Can you work these out from the model? Positions are in its coordinate system, mm. A direction names the side the tool comes from. Round coordinates to 2 decimals unless told otherwise and drop trailing zeros. Loops run counter-clockwise (first coordinate to the right, second up) from the corner with the lowest first, then second, coordinate; pieces in that order, holes last. Notation, with made-up numbers: M 42.5,53 L 65.5,53 A14 ccw 65.5,69 Z; hole C -37.5,29.5 d4. An arc over 180 degrees is marked long. Return JSON: item names as keys, results as strings.
```python
from build123d import *

# Parameters (mm, degrees)
ESQUISSE1_W             = 20
ESQUISSE1_H             = 80
ESQUISSE1_R             = 2.75
BOSS_EXTRU_1_DEPTH      = 5
BOSS_EXTRU_2_DEPTH      = 5
ESQUISSE4_R             = 2.75
BOSS_EXTRU_3_DEPTH      = 25
BOSS_EXTRU_4_DEPTH      = 20
ENL_V_MAT_EXTRU_1_REACH = 78.988
ESQUISSE6_R             = 6
ENL_V_MAT_EXTRU_2_REACH = 103.838
ESQUISSE7_R             = 1.75
ENL_V_MAT_EXTRU_3_REACH = 99.959
ESQUISSE9_R             = 4.5
ENL_V_MAT_EXTRU_4_REACH = 80.753
ESQUISSE10_R            = 2.75


with BuildPart() as part:
    # Esquisse1 → Boss.-Extru.1 (new body)
    with BuildSketch(Plane.XY):
        with Locations((0.415494059, -7.235772358)):
            Rectangle(ESQUISSE1_W, ESQUISSE1_H)
        with Locations((0.415494059, 22.764227642)):
            Circle(ESQUISSE1_R, mode=Mode.SUBTRACT)
        with Locations((0.415494059, -17.235772358)):
            Circle(ESQUISSE1_R, mode=Mode.SUBTRACT)
        with Locations((0.415494059, 2.764227642)):
            Circle(ESQUISSE1_R, mode=Mode.SUBTRACT)
        with Locations((0.415494059, -37.235772358)):
            Circle(ESQUISSE1_R, mode=Mode.SUBTRACT)
    extrude(amount=BOSS_EXTRU_1_DEPTH)

    # Esquisse3 → Boss.-Extru.2 (add)
    with BuildSketch(Plane.XY.offset(5)):
        Polygon((-9.584505941, -47.235772358), (-54.584505941, -47.235772358), (-54.584505941, -42.235772358), (-9.584505941, -27.235772358), align=None)
        Polygon((10.415494059, -47.235772358), (55.415494059, -47.235772358), (55.415494059, -42.235772358), (10.415494059, -27.235772358), align=None)
    extrude(amount=-BOSS_EXTRU_2_DEPTH)

    # Esquisse4 → Boss.-Extru.3 (add)
    with BuildSketch(Plane.XY.offset(5)):
        Polygon((55.415494059, -47.235772358), (55.415494059, -42.235772358), (10.415494059, -27.235772358), (-9.584505941, -27.235772358), (-54.584505941, -42.235772358), (-54.584505941, -47.235772358), align=None)
        with Locations((0.415494059, -37.235772358)):
            Circle(ESQUISSE4_R, mode=Mode.SUBTRACT)
    extrude(amount=BOSS_EXTRU_3_DEPTH)

    # Esquisse5 → Boss.-Extru.4 (add)
    with BuildSketch(Plane.ZY.offset(9.584505941)):
        Polygon((5, -27.235772358), (30, -27.235772358), (5, 32.764227642), align=None)
    extrude(amount=-BOSS_EXTRU_4_DEPTH)

    # Esquisse6 → Enlèv. mat.-Extru.1 (cut, up to next)
    with BuildSketch(Plane(origin=(0, 0, 5), x_dir=(-1, 0, 0), z_dir=(0, 0, -1)), mode=Mode.PRIVATE) as enl_v_mat_extru_1_sk1:
        with Locations((-0.415494059, 2.764227642)):
            Circle(ESQUISSE6_R)
    enl_v_mat_extru_1_tool1 = extrude(enl_v_mat_extru_1_sk1.sketch, amount=-ENL_V_MAT_EXTRU_1_REACH, mode=Mode.PRIVATE) & part.part
    # Esquisse6 → Enlèv. mat.-Extru.1 (cut, up to next)
    with BuildSketch(Plane(origin=(0, 0, 5), x_dir=(-1, 0, 0), z_dir=(0, 0, -1)), mode=Mode.PRIVATE) as enl_v_mat_extru_1_sk2:
        with Locations((-0.415494059, -17.235772358)):
            Circle(ESQUISSE6_R)
    enl_v_mat_extru_1_tool2 = extrude(enl_v_mat_extru_1_sk2.sketch, amount=-ENL_V_MAT_EXTRU_1_REACH, mode=Mode.PRIVATE) & part.part
    # Esquisse6 → Enlèv. mat.-Extru.1 (cut, up to next)
    with BuildSketch(Plane(origin=(0, 0, 5), x_dir=(-1, 0, 0), z_dir=(0, 0, -1)), mode=Mode.PRIVATE) as enl_v_mat_extru_1_sk3:
        with Locations((-0.415494059, 22.764227642)):
            Circle(ESQUISSE6_R)
    enl_v_mat_extru_1_tool3 = extrude(enl_v_mat_extru_1_sk3.sketch, amount=-ENL_V_MAT_EXTRU_1_REACH, mode=Mode.PRIVATE) & part.part
    # Esquisse6 → Enlèv. mat.-Extru.1 (cut, up to next)
    with BuildSketch(Plane(origin=(0, 0, 5), x_dir=(-1, 0, 0), z_dir=(0, 0, -1)), mode=Mode.PRIVATE) as enl_v_mat_extru_1_sk4:
        with Locations((-0.415494059, -37.235772358)):
            Circle(ESQUISSE6_R)
    enl_v_mat_extru_1_tool4 = extrude(enl_v_mat_extru_1_sk4.sketch, amount=-ENL_V_MAT_EXTRU_1_REACH, mode=Mode.PRIVATE) & part.part
    add(enl_v_mat_extru_1_tool1.solids().sort_by_distance((0.415494, 2.764228, 5))[0], mode=Mode.SUBTRACT)
    add(enl_v_mat_extru_1_tool2.solids().sort_by_distance((0.415494, -17.235772, 5))[0], mode=Mode.SUBTRACT)
    add(enl_v_mat_extru_1_tool3.solids().sort_by_distance((0.415494, 22.764228, 5))[0], mode=Mode.SUBTRACT)
    add(enl_v_mat_extru_1_tool4.solids().sort_by_distance((0.415494, -37.235772, 5))[0], mode=Mode.SUBTRACT)

    # Esquisse7 → Enlèv. mat.-Extru.2 (cut, up to next)
    with BuildSketch(Plane.XZ.offset(47.235772358), mode=Mode.PRIVATE) as enl_v_mat_extru_2_sk1:
        with Locations(Location((-42.084505941, 25, 0), (0, 0, 270))):
            Circle(ESQUISSE7_R)
    enl_v_mat_extru_2_tool1 = extrude(enl_v_mat_extru_2_sk1.sketch, amount=-ENL_V_MAT_EXTRU_2_REACH, mode=Mode.PRIVATE) & part.part
    # Esquisse7 → Enlèv. mat.-Extru.2 (cut, up to next)
    with BuildSketch(Plane.XZ.offset(47.235772358), mode=Mode.PRIVATE) as enl_v_mat_extru_2_sk2:
        with Locations(Location((-22.084505941, 25, 0), (0, 0, 270))):
            Circle(ESQUISSE7_R)
    enl_v_mat_extru_2_tool2 = extrude(enl_v_mat_extru_2_sk2.sketch, amount=-ENL_V_MAT_EXTRU_2_REACH, mode=Mode.PRIVATE) & part.part
    # Esquisse7 → Enlèv. mat.-Extru.2 (cut, up to next)
    with BuildSketch(Plane.XZ.offset(47.235772358), mode=Mode.PRIVATE) as enl_v_mat_extru_2_sk3:
        with Locations(Location((-22.084505941, 5, 0), (0, 0, 270))):
            Circle(ESQUISSE7_R)
    enl_v_mat_extru_2_tool3 = extrude(enl_v_mat_extru_2_sk3.sketch, amount=-ENL_V_MAT_EXTRU_2_REACH, mode=Mode.PRIVATE) & part.part
    # Esquisse7 → Enlèv. mat.-Extru.2 (cut, up to next)
    with BuildSketch(Plane.XZ.offset(47.235772358), mode=Mode.PRIVATE) as enl_v_mat_extru_2_sk4:
        with Locations(Location((-42.084505941, 5, 0), (0, 0, 270))):
            Circle(ESQUISSE7_R)
    enl_v_mat_extru_2_tool4 = extrude(enl_v_mat_extru_2_sk4.sketch, amount=-ENL_V_MAT_EXTRU_2_REACH, mode=Mode.PRIVATE) & part.part
    # Esquisse7 → Enlèv. mat.-Extru.2 (cut, up to next)
    with BuildSketch(Plane.XZ.offset(47.235772358), mode=Mode.PRIVATE) as enl_v_mat_extru_2_sk5:
        with Locations(Location((42.915494059, 25, 0), (0, 0, 270))):
            Circle(ESQUISSE7_R)
    enl_v_mat_extru_2_tool5 = extrude(enl_v_mat_extru_2_sk5.sketch, amount=-ENL_V_MAT_EXTRU_2_REACH, mode=Mode.PRIVATE) & part.part
    # Esquisse7 → Enlèv. mat.-Extru.2 (cut, up to next)
    with BuildSketch(Plane.XZ.offset(47.235772358), mode=Mode.PRIVATE) as enl_v_mat_extru_2_sk6:
        with Locations(Location((42.915494059, 5, 0), (0, 0, 270))):
            Circle(ESQUISSE7_R)
    enl_v_mat_extru_2_tool6 = extrude(enl_v_mat_extru_2_sk6.sketch, amount=-ENL_V_MAT_EXTRU_2_REACH, mode=Mode.PRIVATE) & part.part
    # Esquisse7 → Enlèv. mat.-Extru.2 (cut, up to next)
    with BuildSketch(Plane.XZ.offset(47.235772358), mode=Mode.PRIVATE) as enl_v_mat_extru_2_sk7:
        with Locations(Location((22.915494059, 5, 0), (0, 0, 270))):
            Circle(ESQUISSE7_R)
    enl_v_mat_extru_2_tool7 = extrude(enl_v_mat_extru_2_sk7.sketch, amount=-ENL_V_MAT_EXTRU_2_REACH, mode=Mode.PRIVATE) & part.part
    # Esquisse7 → Enlèv. mat.-Extru.2 (cut, up to next)
    with BuildSketch(Plane.XZ.offset(47.235772358), mode=Mode.PRIVATE) as enl_v_mat_extru_2_sk8:
        with Locations(Location((22.915494059, 25, 0), (0, 0, 270))):
            Circle(ESQUISSE7_R)
    enl_v_mat_extru_2_tool8 = extrude(enl_v_mat_extru_2_sk8.sketch, amount=-ENL_V_MAT_EXTRU_2_REACH, mode=Mode.PRIVATE) & part.part
    add(enl_v_mat_extru_2_tool1.solids().sort_by_distance((-42.084506, -47.235772, 25))[0], mode=Mode.SUBTRACT)
    add(enl_v_mat_extru_2_tool2.solids().sort_by_distance((-22.084506, -47.235772, 25))[0], mode=Mode.SUBTRACT)
    add(enl_v_mat_extru_2_tool3.solids().sort_by_distance((-22.084506, -47.235772, 5))[0], mode=Mode.SUBTRACT)
    add(enl_v_mat_extru_2_tool4.solids().sort_by_distance((-42.084506, -47.235772, 5))[0], mode=Mode.SUBTRACT)
    add(enl_v_mat_extru_2_tool5.solids().sort_by_distance((42.915494, -47.235772, 25))[0], mode=Mode.SUBTRACT)
    add(enl_v_mat_extru_2_tool6.solids().sort_by_distance((42.915494, -47.235772, 5))[0], mode=Mode.SUBTRACT)
    add(enl_v_mat_extru_2_tool7.solids().sort_by_distance((22.915494, -47.235772, 5))[0], mode=Mode.SUBTRACT)
    add(enl_v_mat_extru_2_tool8.solids().sort_by_distance((22.915494, -47.235772, 25))[0], mode=Mode.SUBTRACT)

    # Esquisse9 → Enlèv. mat.-Extru.3 (cut, up to next)
    with BuildSketch(Plane(origin=(0, -42.235772358, 0), x_dir=(-1, 0, 0), z_dir=(0, -1, 0)), mode=Mode.PRIVATE) as enl_v_mat_extru_3_sk1:
        with Locations(Location((42.084505941, -25, 0), (0, 0, 90))):
            Circle(ESQUISSE9_R)
    enl_v_mat_extru_3_tool1 = extrude(enl_v_mat_extru_3_sk1.sketch, amount=-ENL_V_MAT_EXTRU_3_REACH, mode=Mode.PRIVATE) & part.part
    # Esquisse9 → Enlèv. mat.-Extru.3 (cut, up to next)
    with BuildSketch(Plane(origin=(0, -42.235772358, 0), x_dir=(-1, 0, 0), z_dir=(0, -1, 0)), mode=Mode.PRIVATE) as enl_v_mat_extru_3_sk2:
        with Locations(Location((22.084505941, -25, 0), (0, 0, 90))):
            Circle(ESQUISSE9_R)
    enl_v_mat_extru_3_tool2 = extrude(enl_v_mat_extru_3_sk2.sketch, amount=-ENL_V_MAT_EXTRU_3_REACH, mode=Mode.PRIVATE) & part.part
    # Esquisse9 → Enlèv. mat.-Extru.3 (cut, up to next)
    with BuildSketch(Plane(origin=(0, -42.235772358, 0), x_dir=(-1, 0, 0), z_dir=(0, -1, 0)), mode=Mode.PRIVATE) as enl_v_mat_extru_3_sk3:
        with Locations(Location((22.084505941, -5, 0), (0, 0, 90))):
            Circle(ESQUISSE9_R)
    enl_v_mat_extru_3_tool3 = extrude(enl_v_mat_extru_3_sk3.sketch, amount=-ENL_V_MAT_EXTRU_3_REACH, mode=Mode.PRIVATE) & part.part
    # Esquisse9 → Enlèv. mat.-Extru.3 (cut, up to next)
    with BuildSketch(Plane(origin=(0, -42.235772358, 0), x_dir=(-1, 0, 0), z_dir=(0, -1, 0)), mode=Mode.PRIVATE) as enl_v_mat_extru_3_sk4:
        with Locations(Location((42.084505941, -5, 0), (0, 0, 90))):
            Circle(ESQUISSE9_R)
    enl_v_mat_extru_3_tool4 = extrude(enl_v_mat_extru_3_sk4.sketch, amount=-ENL_V_MAT_EXTRU_3_REACH, mode=Mode.PRIVATE) & part.part
    # Esquisse9 → Enlèv. mat.-Extru.3 (cut, up to next)
    with BuildSketch(Plane(origin=(0, -42.235772358, 0), x_dir=(-1, 0, 0), z_dir=(0, -1, 0)), mode=Mode.PRIVATE) as enl_v_mat_extru_3_sk5:
        with Locations(Location((-22.915494059, -25, 0), (0, 0, 90))):
            Circle(ESQUISSE9_R)
    enl_v_mat_extru_3_tool5 = extrude(enl_v_mat_extru_3_sk5.sketch, amount=-ENL_V_MAT_EXTRU_3_REACH, mode=Mode.PRIVATE) & part.part
    # Esquisse9 → Enlèv. mat.-Extru.3 (cut, up to next)
    with BuildSketch(Plane(origin=(0, -42.235772358, 0), x_dir=(-1, 0, 0), z_dir=(0, -1, 0)), mode=Mode.PRIVATE) as enl_v_mat_extru_3_sk6:
        with Locations(Location((-42.915494059, -25, 0), (0, 0, 90))):
            Circle(ESQUISSE9_R)
    enl_v_mat_extru_3_tool6 = extrude(enl_v_mat_extru_3_sk6.sketch, amount=-ENL_V_MAT_EXTRU_3_REACH, mode=Mode.PRIVATE) & part.part
    # Esquisse9 → Enlèv. mat.-Extru.3 (cut, up to next)
    with BuildSketch(Plane(origin=(0, -42.235772358, 0), x_dir=(-1, 0, 0), z_dir=(0, -1, 0)), mode=Mode.PRIVATE) as enl_v_mat_extru_3_sk7:
        with Locations(Location((-42.915494059, -5, 0), (0, 0, 90))):
            Circle(ESQUISSE9_R)
    enl_v_mat_extru_3_tool7 = extrude(enl_v_mat_extru_3_sk7.sketch, amount=-ENL_V_MAT_EXTRU_3_REACH, mode=Mode.PRIVATE) & part.part
    # Esquisse9 → Enlèv. mat.-Extru.3 (cut, up to next)
    with BuildSketch(Plane(origin=(0, -42.235772358, 0), x_dir=(-1, 0, 0), z_dir=(0, -1, 0)), mode=Mode.PRIVATE) as enl_v_mat_extru_3_sk8:
        with Locations(Location((-22.915494059, -5, 0), (0, 0, 90))):
            Circle(ESQUISSE9_R)
    enl_v_mat_extru_3_tool8 = extrude(enl_v_mat_extru_3_sk8.sketch, amount=-ENL_V_MAT_EXTRU_3_REACH, mode=Mode.PRIVATE) & part.part
    add(enl_v_mat_extru_3_tool1.solids().sort_by_distance((-42.084506, -42.235772, 25))[0], mode=Mode.SUBTRACT)
    add(enl_v_mat_extru_3_tool2.solids().sort_by_distance((-22.084506, -42.235772, 25))[0], mode=Mode.SUBTRACT)
    add(enl_v_mat_extru_3_tool3.solids().sort_by_distance((-22.084506, -42.235772, 5))[0], mode=Mode.SUBTRACT)
    add(enl_v_mat_extru_3_tool4.solids().sort_by_distance((-42.084506, -42.235772, 5))[0], mode=Mode.SUBTRACT)
    add(enl_v_mat_extru_3_tool5.solids().sort_by_distance((22.915494, -42.235772, 25))[0], mode=Mode.SUBTRACT)
    add(enl_v_mat_extru_3_tool6.solids().sort_by_distance((42.915494, -42.235772, 25))[0], mode=Mode.SUBTRACT)
    add(enl_v_mat_extru_3_tool7.solids().sort_by_distance((42.915494, -42.235772, 5))[0], mode=Mode.SUBTRACT)
    add(enl_v_mat_extru_3_tool8.solids().sort_by_distance((22.915494, -42.235772, 5))[0], mode=Mode.SUBTRACT)

    # Esquisse10 → Enlèv. mat.-Extru.4 (cut, up to next)
    with BuildSketch(Plane.XY.offset(30), mode=Mode.PRIVATE) as enl_v_mat_extru_4_sk1:
        with Locations((14.415494059, -42.235772358)):
            Circle(ESQUISSE10_R)
    enl_v_mat_extru_4_tool1 = extrude(enl_v_mat_extru_4_sk1.sketch, amount=-ENL_V_MAT_EXTRU_4_REACH, mode=Mode.PRIVATE) & part.part
    # Esquisse10 → Enlèv. mat.-Extru.4 (cut, up to next)
    with BuildSketch(Plane.XY.offset(30), mode=Mode.PRIVATE) as enl_v_mat_extru_4_sk2:
        with Locations((31.415494059, -42.235772358)):
            Circle(ESQUISSE10_R)
    enl_v_mat_extru_4_tool2 = extrude(enl_v_mat_extru_4_sk2.sketch, amount=-ENL_V_MAT_EXTRU_4_REACH, mode=Mode.PRIVATE) & part.part
    add(enl_v_mat_extru_4_tool1.solids().sort_by_distance((14.415494, -42.235772, 30))[0], mode=Mode.SUBTRACT)
    add(enl_v_mat_extru_4_tool2.solids().sort_by_distance((31.415494, -42.235772, 30))[0], mode=Mode.SUBTRACT)


solid = part.part
```
Q1. If I drill on line 1 along X through (y, z) = (-46.05, 25); line 2 along X through (y, z) = (-37.5, 24.5); line 3 along X through (y, z) = (-38.6, 25), over which ranges is the centre line in solid material (lowest first)?
Results:
{"line 1": "x = -54.58 to -43.83, -40.33 to -23.83, -20.33 to 21.17, 24.67 to 41.17, 44.67 to 55.42", "line 2": "x = -37.61 to -26.56, -17.61 to -5.58, 6.41 to 18.44, 27.39 to 38.44", "line 3": "x = -37.58 to -26.58, -17.58 to -5.43, 6.26 to 18.42, 27.42 to 38.42"}
Q2. Thinking about a two-plate mould opening in Y: for faces 1 (the cylindrical face through (-2.33, 2.89, 2.46)), 2 (the flat face through (-6.391, 2.344, 17.675)), 3 (the cylindrical face through (-0.18, -39.92, 2.46)), 4 (the flat face through (0, -47.236, 15)), which applies, pulls with the +Y half, pulls with the -Y half, needs draft (parallel to the pull), parting line crosses it, or undercut?
Results:
{"face 1": "undercut", "face 2": "pulls with the +Y half", "face 3": "undercut", "face 4": "pulls with the -Y half"}
Q3. On a 3-axis mill with a long thin cutter (end or side, diameter ignored), from which of +Z, -Z, +X, -X, +Y, -Y can I reach the whole of each face in a straight line? I mean faces 5 (the flat face through (10.415, -3, 11)), 6 (the cylindrical face through (44.65, -44.77, 5.23)), 7 (the flat face through (-2.2, 21.5, 5)), 8 (the cylindrical face through (38.523, -40.058, 5.976)). Say none if no direction works.
Results:
{"face 5": "+Z, -Z, +X, +Y", "face 6": "+Y, -Y", "face 7": "+Z", "face 8": "+Y"}
Q4. Suppose I cut it at C-C, the plane z = 16.25. Please give me the cut outline in (x, y), plus the area to 3 significant figures.
Results:
{"outline": "M -54.58,-47.24 L 55.42,-47.24 L 55.42,-42.24 L 10.42,-27.24 L 10.42,5.76 L 5.61,5.76 A6 cw long -4.78,5.76 L -9.58,5.76 L -9.58,-27.24 L -54.58,-42.24 Z; hole C 0.42,-37.24 d12; hole C 0.42,-17.24 d12; hole C 14.42,-42.24 d5.5; hole C 31.42,-42.24 d5.5", "area": "1,820 mm2"}
Q5. Suppose I cut it at B-B, the plane y = -13. Please give me the cut outline in (x, z) (1 decimal).
Results:
{"outline": "M -9.6,0 L 10.4,0 L 10.4,24.1 L 4.7,24.1 L 4.7,5 L -3.8,5 L -3.8,24.1 L -9.6,24.1 Z"}
Q6. I'm going to push flat-ended pins straight in: pin 1 Ø12 at (x, z) = (28, 15) entering from +Y; pin 2 Ø4 at (y, z) = (19, 3.5) entering from +X; pin 3 Ø4.5 at (x, z) = (43, 4) entering from +Y. Where does each tip first touch, or does it pass through?
Results:
{"pin 1": "stops at y = -31.1", "pin 2": "stops at x = 10.42", "pin 3": "stops at y = -42.24"}
Q7. Suppose I cut it at D-D, the plane x = -29. Please give me the cut outline in (y, z), plus the area to 3 significant figures.
Results:
{"outline": "M -47.24,0 L -33.71,0 L -33.71,30 L -47.24,30 Z", "area": "406 mm2"}
Q8. Suppose I cut it at A-A, the plane x = -45. Please give me the cut outline in (y, z), plus the area to 3 significant figures.
Results:
{"outline": "M -47.24,0 L -39.04,0 L -39.04,1.57 L -42.24,1.57 L -42.24,8.43 L -39.04,8.43 L -39.04,21.57 L -42.24,21.57 L -42.24,28.43 L -39.04,28.43 L -39.04,30 L -47.24,30 Z", "area": "202 mm2"}
